Can you work these out from the model? Positions are in its coordinate system, mm. A direction names the side the tool comes from. Give positions to 0.01 mm unless a question says otherwise; leave off trailing zeros. Loops run counter-clockwise (first coordinate to the right, second up) from the corner with the lowest first, then second, coordinate; pieces in that order, holes last. Notation, with made-up numbers: (65.5, 42) - (76.5, 42) arc R18 ccw to (76.5, 60) - close; hole circle Ø9 at (41.5, 28). An arc over 180 degrees is marked (long way). Answer in a Markdown table with one row per item.
from build123d import *

# Parameters (mm, degrees)
F0_W            = 12.5
F0_H            = 2.5
F2_W            = 30
F2_H            = 5
F3_DEPTH        = 4
F3_TAPER        = -3
F3_COPIES_COUNT = 3
F3_COPIES_ANGLE = 120
F4_SIZE         = 2


# Not quite as in the source:
# - a pattern or mirror of a feature is missing from the dataset's text; its kind, count and spacing are read off the source's solid


with BuildPart() as f1:
    # F0 (on Front) → F1 (revolve)
    with BuildSketch(Plane.XZ):
        Polygon((10, 0), (8, 0), (8, -8), (0, -8), (0, -10), (8, -10), (10, -8), align=None)
        with BuildLine():
            Line((8, -10), (0, -10))
            Line((0, -10), (0, -45.5))
            Line((0, -45.5), (12.5, -45.5))
            add(Edge.make_bspline(
                [(8, -10), (5.9036325589, -11.9965153095), (1.0129290603, -16.5253438832), (13.2882333552, -27.2092652156), (4.5052088966, -39.5192070851), (9.2502525397, -41.9720056367), (8.9567015183, -44.5926383173), (11.3466967049, -45.1906230325), (12.5, -45.5)],
                knots=[0, 0, 0, 0, 0.1843856525, 0.4236571978, 0.6554974409, 0.7819959318, 0.8777293444, 1, 1, 1, 1], degree=3))
        make_face()
        with Locations((6.25, -46.75)):
            Rectangle(F0_W, F0_H)
    revolve(axis=Axis((0, 0, -24), (0, 0, -1)))

    # F2 (on face) → F3 (cut)
    with BuildSketch(Plane.XY):
        Rectangle(F2_W, F2_H)
    f3 = extrude(amount=-F3_DEPTH, taper=F3_TAPER, mode=Mode.SUBTRACT)

    # F3_copies: F3 ×3 about axis
    f3_copies_axis = Axis((0, 0, 0), (0, 0, 1))
    for i in range(1, F3_COPIES_COUNT):
        add(f3.rotate(f3_copies_axis, i * F3_COPIES_ANGLE / (F3_COPIES_COUNT - 1)), mode=Mode.SUBTRACT)

    # F4
    f4_edges = [f1.edges().sort_by_distance(p)[0] for p in [
        (-8, 0, -8),
    ]]
    chamfer(f4_edges, length=F4_SIZE)


solid = f1.part
Q1. Imagine slicing it at B-B, the plane x = 9. Count the separate pieces of the cut face and the enclosed holes in it, and give its area (3 significant figures).
Checked values:
| item | result |
|---|---|
| separate pieces | 3 |
| enclosed holes | 0 |
| area | 139 mm² |
Q2. On a 3-axis mill with a long thin cutter (end or side, diameter ignored), from which of +Z, -Z, +X, -X, +Y, -Y can I reach the whole of each face in a straight line? I mean faces 1 (the face through (7.39, 3.06, -3.71)), 2 (the face through (-9, 0, -4)), 3 (the face through (-4, -8, -4)). Say none if no direction works.
Checked values:
| item | result |
|---|---|
| face 1 | +Z |
| face 2 | +X, -X |
| face 3 | none |
Q3. If we mould it in two halves opening along Z, with no side actions, what happens to faces 4 (the face through (-8, 4, 0)), 5 (the face through (11.923, -3.755, -46.732)), 6 (the face through (-1.06, -8.06, -9.87))? For each: released by +Z, released by -Z, zero draft, split by the parting line, or undercut.
Checked values:
| item | result |
|---|---|
| face 4 | released by +Z |
| face 5 | zero draft |
| face 6 | undercut |
Q4. Imagine slicing it at A-A, the plane z = -9.5. Write out the boundary of the cut face in (x, y).
Checked values:
| item | result |
|---|---|
| outline | circle Ø17 at (0, 0) |
Q5. If I drill on line 1 (Y direction, x = 0, z = -1.5); line 2 (Z direction, x = -6, y = 2.25); line 3 (Y direction, x = 3.5, z = -11.5), over which ranges is the centre line in solid material (lowest first)? Write a range as [from, to].
Checked values:
| item | result |
|---|---|
| line 1 | y = [-10, -8], [8, 10] |
| line 2 | z = [-48, -21.17], [-11.55, -7.59] |
| line 3 | y = [-5.43, 5.43] |
Q6. For pin 1 (2.5 mm diameter, centred on x = 5, y = -6.5, fed in from +Z); pin 2 (12 mm diameter, centred on y = 10, z = -20.5, fed in from -X); pin 3 (6 mm diameter, centred on x = 8.5, z = -40.5, fed in from +Y), each with a flat end and sliding along its axis, tell me the tip position at first contact or that it passes through.
Checked values:
| item | result |
|---|---|
| pin 1 | stops at z = -4 |
| pin 2 | stops at x = -6.28 |
| pin 3 | stops at y = 6.29 |
